Geometry check sheet. Reference: the model listing, model coordinates, mm. A direction names the side the tool comes from. Coordinates: 2 decimals unless noted, no trailing zeros. Loops run counter-clockwise (first coordinate to the right, second up) from the corner with the lowest first, then second, coordinate; pieces in that order, holes last.
from build123d import *

# Parameters (mm, degrees)
F0_W     = 75
F0_H     = 50
F1_DEPTH = 25
F3_DEPTH = 25


with BuildPart() as f1:
    # F0 (on Front) → F1 (new body)
    with BuildSketch(Plane.XZ):
        with Locations((-2.86842, 7.68421)):
            Rectangle(F0_W, F0_H)
    extrude(amount=F1_DEPTH)

    # F2 (on Front) → F3 (cut)
    with BuildSketch(Plane.XZ):
        Polygon((-19.781306, 22.144739), (-22.781306, 22.144739), (-22.781306, 7.144739), (-2.781306, 7.144739), (-2.781306, 12.144739), (-19.781306, 12.144739), align=None)
    extrude(amount=F3_DEPTH, mode=Mode.SUBTRACT)


solid = f1.part
(1) Sectioned sample at B-B on x = -8. Record the cut outline in (y, z).
Findings:
outline: (-25, -17.32) - (0, -17.32) - (0, 7.14) - (-25, 7.14) - close; (-25, 12.14) - (0, 12.14) - (0, 32.68) - (-25, 32.68) - close
(2) Scan lines: L1, parallel to Z at x = -12, y = -18; L2, parallel to X at y = -5.25, z = 10; L3, parallel to Z at x = -20.5, y = -6.5. Record each from-to range of solid material in increasing order.
Findings:
L1: z = -17.32 to 7.14, 12.14 to 32.68
L2: x = -40.37 to -22.78, -2.78 to 34.63
L3: z = -17.32 to 7.14, 22.14 to 32.68
(3) Sectioned sample at A-A on z = 10. Record the cut outline in (x, y), and give its area (4 significant figures).
Findings:
outline: (-40.37, -25) - (-22.78, -25) - (-22.78, 0) - (-40.37, 0) - close; (-2.78, -25) - (34.63, -25) - (34.63, 0) - (-2.78, 0) - close
area: 1,375 mm2
(4) Access from +Z, -Z, +X, -X, +Y, -Y to the whole of each face (thin tool, end or side, straight path). Record for faces 4 (the flat face through (-3, -25, 2)), 5 (the flat face through (-11, -12, 12.145)).
Findings:
face 4: +Z, -Z, +X, -X, -Y
face 5: +Y, -Y
(5) Sectioned sample at C-C on y = -2.5. Record the cut outline in (x, z), and give its area (3 significant figures).
Findings:
outline: (-40.37, -17.32) - (34.63, -17.32) - (34.63, 32.68) - (-40.37, 32.68) - close; hole (-22.78, 7.14) - (-2.78, 7.14) - (-2.78, 12.14) - (-19.78, 12.14) - (-19.78, 22.14) - (-22.78, 22.14) - close
area: 3,620 mm2
(6) Draft check along X on faces 1 (the flat face through (34.632, -12, 7)), 2 (the flat face through (-22.781, -12, 15)), 3 (the flat face through (-3, -12, -17.316)). Enter one of: +X half, -X half, draft (parallel to the pull), parting line (faces both ways), or undercut.
Findings:
face 1: +X half
face 2: undercut
face 3: draft
